from build123d import *

# Parameters (mm, degrees)
SKETCH1_R                           = 22.225
SKETCH1_R_2                         = 12.7
BOSS_EXTRUDE1_DEPTH                 = 50.8
SKETCH2_R                           = 3.175
CUT_EXTRUDE1_DEPTH                  = 60.737268518
CUT_EXTRUDE1_DEPTH_BACK             = 60.737268518
F_5_16_0_3125_DIAMETER_HOLE1_REACH  = 59.326
F_5_16_0_3125_DIAMETER_HOLE1_BORE_R = 3.96875
CUT_EXTRUDE3_REACH                  = 61.737
SKETCH6_W                           = 6.35
SKETCH6_H                           = 3.175


with BuildPart() as part:
    # Sketch1 → Boss-Extrude1 (new body)
    with BuildSketch(Plane(origin=(0, 0, 0), x_dir=(1, 0, 0), z_dir=(0, 1, 0))):
        with Locations(Location((0, 0, 0), (0, 0, 270))):
            Circle(SKETCH1_R)
        with Locations(Location((0, 0, 0), (0, 0, 270))):
            Circle(SKETCH1_R_2, mode=Mode.SUBTRACT)
    extrude(amount=BOSS_EXTRUDE1_DEPTH)

    # Sketch2 → Cut-Extrude1 (cut, two sides)
    with BuildSketch(Plane.XY) as cut_extrude1_sk:
        with Locations((0, 9.525)):
            Circle(SKETCH2_R)
    extrude(amount=CUT_EXTRUDE1_DEPTH, mode=Mode.SUBTRACT)
    extrude(cut_extrude1_sk.sketch, amount=-CUT_EXTRUDE1_DEPTH_BACK, mode=Mode.SUBTRACT)

    # 5/16 (0.3125) Diameter Hole1 bore (on position points) → 5/16 (0.3125) Diameter Hole1 (cut, up to next)
    with BuildSketch(Plane(origin=(0, 28.575, 22.225), x_dir=(1, 0, 0), z_dir=(0, 0, 1)), mode=Mode.PRIVATE) as f_5_16_0_3125_diameter_hole1_sk1:
        Circle(F_5_16_0_3125_DIAMETER_HOLE1_BORE_R)
    f_5_16_0_3125_diameter_hole1_tool1 = extrude(f_5_16_0_3125_diameter_hole1_sk1.sketch, amount=-F_5_16_0_3125_DIAMETER_HOLE1_REACH, mode=Mode.PRIVATE) & part.part
    add(f_5_16_0_3125_diameter_hole1_tool1.solids().sort_by_distance((0, 28.575, 22.225))[0], mode=Mode.SUBTRACT)

    # Cut-Extrude3: up to this face of the body (flat: up to its plane)
    cut_extrude3_end = Plane(part.part.faces().sort_by_distance((0, 0, -21.596382072))[0])
    # Sketch6 → Cut-Extrude3 (cut, up to the picked face)
    with BuildSketch(Plane(origin=(0, 50.8, 0), x_dir=(1, 0, 0), z_dir=(0, 1, 0)), mode=Mode.PRIVATE) as cut_extrude3_sk1:
        with Locations((0, -13.884222124)):
            Rectangle(SKETCH6_W, SKETCH6_H)
    cut_extrude3_tool1 = split(extrude(cut_extrude3_sk1.sketch, amount=-CUT_EXTRUDE3_REACH, mode=Mode.PRIVATE), bisect_by=cut_extrude3_end, keep=Keep.BOTH, mode=Mode.PRIVATE)
    add(cut_extrude3_tool1.solids().sort_by(Axis((0, 50.8, 13.884222), (0, -1, 0)))[0], mode=Mode.SUBTRACT)


solid = part.part
Can you work these out from the model? Positions are in its coordinate system, mm. A direction names the side the tool comes from. Coordinates: 2 decimals unless noted, no trailing zeros. Loops run counter-clockwise (first coordinate to the right, second up) from the corner with the lowest first, then second, coordinate; pieces in that order, holes last. Notation, with made-up numbers: (21, 66) - (42, 66) arc R32 ccw to (42, 100) - close; hole circle Ø4 at (19, 45.5). An arc over 180 degrees is marked (long way). Answer as a JSON object with one key per item and string values. Group by question number.
Item 1: If we section it at B-B (x = 0): List the corners of the cut face in (y, z) for me (3 decimals).
Item 2: If we section it at D-D (x = 12): List the corners of the cut face in (y, z) for me.
Item 3: For pin 1 (8 mm diameter, centred on y = 12, z = -8, fed in from -X); pin 2 (3 mm diameter, centred on x = -12, y = 43.5, fed in from -Z); pin 3 (1 mm diameter, centred on x = -11, y = 14.5, fed in from +Z), each with a flat end and sliding along its axis, tell me the tip position at first contact or that it passes through.
Item 4: If we section it at A-A (z = 0): List the corners of the cut face in (x, y) for me (3 decimals).
Item 5: If I drill on L1, parallel to Y at x = 0, z = 19; L2, parallel to Z at x = 0, y = 23 (3 decimals); L3, parallel to Z at x = -11.5, y = 19.5, over which ranges is the centre line in solid material (lowest first)? Write a range as from..to.
Item 6: If we section it at C-C (y = 5): List the corners of the cut face in (x, z) for me (3 decimals), plus the area to 3 significant figures.
Item 7: On a 3-axis mill with a long thin cutter (end or side, diameter ignored), from which of +Z, -Z, +X, -X, +Y, -Y can I reach the whole of each face in a straight line? I mean faces 4 (the face through (3.785, 29.767, 18.344)), 5 (the face through (-3.175, 41, 14)), 6 (the face through (1.71, 12.2, 18.8)). Say none if no direction works.
Item 8: If we mould it in two halves opening along X, with no side actions, what happens to faces 1 (the face through (6.676, 25.044, 21.199)), 2 (the face through (-10, 50.8, 10)), 3 (the face through (0, 4, 15.472))? For each: released by +X, released by -X, zero draft, split by the parting line, or undercut.
Returned:
{
 "1": {"outline": "(0, -22.225) - (6.35, -22.225) - (6.35, -12.7) - (0, -12.7) - close; (0, 15.472) - (6.35, 15.472) - (6.35, 22.225) - (0, 22.225) - close; (12.7, -22.225) - (50.8, -22.225) - (50.8, -12.7) - (12.7, -12.7) - close; (12.7, 15.472) - (24.606, 15.472) - (24.606, 22.225) - (12.7, 22.225) - close; (32.544, 15.472) - (50.8, 15.472) - (50.8, 22.225) - (32.544, 22.225) - close"},
 "2": {"outline": "(0, -18.71) - (50.8, -18.71) - (50.8, -4.16) - (0, -4.16) - close; (0, 4.16) - (50.8, 4.16) - (50.8, 18.71) - (0, 18.71) - close"},
 "3": {"pin 1": "stops at x = -21.86", "pin 2": "stops at z = -19.59", "pin 3": "stops at z = 19.59"},
 "4": {"outline": "(-22.225, 0) - (-12.7, 0) - (-12.7, 50.8) - (-22.225, 50.8) - close; (12.7, 0) - (22.225, 0) - (22.225, 50.8) - (12.7, 50.8) - close"},
 "5": {"L1": "y = 0..6.35, 12.7..24.61, 32.54..50.8", "L2": "z = -22.225..-12.7, 15.472..22.225", "L3": "z = -19.02..-5.39, 5.39..19.02"},
 "6": {"outline": "circle Ø44.45 at (0, 0); hole (-3.175, 12.297) arc R12.7 ccw (long way) to (3.175, 12.297) - (3.175, 15.472) - (-3.175, 15.472) - close", "area": "1,030 mm²"},
 "7": {"face 4": "+Z", "face 5": "+Y, -Y", "face 6": "+Z, -Z"},
 "8": {"face 1": "split by the parting line", "face 2": "zero draft", "face 3": "undercut"}
}
